Check sheet for the modelled part. Datum: model origin and axes. Units: mm. Face numbers are marked on the shaded views. A direction names the side the tool comes from. Give positions to 0.01 mm unless a question says otherwise; leave off trailing zeros. Order: outer loops, then holes, each group sorted by start corner. A loop starts at its lowest first (then second) coordinate and runs counter-clockwise, first axis right, second up.
Item 1: Sectioned sample at A-A on x = 0. Record the boundary of the cut face in (y, z), and give its area (3 significant figures).
Item 2: Material ranges on line 1 along Z through (x, y) = (-0.95, -0.6); line 2 along Z through (x, y) = (-2.05, 0.45); line 3 along X through (y, z) = (0.9, 19), recorded low to high.
Item 3: Gauge pin test, flat ends, axial feed: P1, Ø0.8, axis at x = 0, y = 0, coming from the -Z side; P2, Ø1.5, axis at x = -1, z = 7, coming from the -Y side. Record the tip position at first contact, or that the pin passes through.
Item 4: Access from +Z, -Z, +X, -X, +Y, -Y to the whole of each face (thin tool, end or side, straight path). Record for the marked faces 1 and 2.
Item 5: Sectioned sample at B-B on z = 12. Record the boundary of the cut face in (x, y).
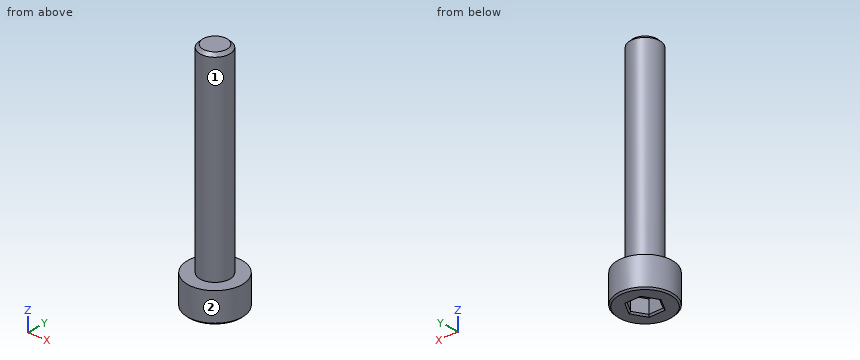
from build123d import *

# Parameters (mm, degrees)
F3_R     = 2.75
F4_DEPTH = 3
F6_DEPTH = 1.5
F7_R     = 1.5
F8_DEPTH = 20
F9_SIZE  = 0.15
F10_SIZE = 0.3


with BuildPart() as f4:
    # F3 (on Top) → F4 (new body)
    with BuildSketch(Plane.XY):
        Circle(F3_R)
    extrude(amount=F4_DEPTH)

    # F5 (on face) → F6 (cut)
    with BuildSketch(Plane(origin=(0, 0, 0), x_dir=(1, 0, 0), z_dir=(0, 0, -1))):
        Polygon((0.7216878365, 1.25), (-0.7216878365, 1.25), (-1.443375673, 0), (-0.7216878365, -1.25), (0.7216878365, -1.25), (1.443375673, 0), align=None)
    extrude(amount=-F6_DEPTH, mode=Mode.SUBTRACT)

    # F7 (on face) → F8 (join)
    with BuildSketch(Plane.XY.offset(3)):
        Circle(F7_R)
    extrude(amount=F8_DEPTH)

    # F9
    f9_edges = [f4.edges().sort_by_distance(p)[0] for p in [
        (-2.75, 0, 0),
        (0, -1.25, 0),
        (1.082532, -0.625, 0),
        (1.082532, 0.625, 0),
        (0, 1.25, 0),
        (-1.082532, -0.625, 0),
        (-1.082532, 0.625, 0),
    ]]
    chamfer(f9_edges, length=F9_SIZE)

    # F10
    f10_edges = [f4.edges().sort_by_distance(p)[0] for p in [
        (-1.5, 0, 23),
    ]]
    chamfer(f10_edges, length=F10_SIZE)


solid = f4.part
Report:
1. outline: (-2.75, 0.15) - (-2.6, 0) - (-1.4, 0) - (-1.25, 0.15) - (-1.25, 1.5) - (1.25, 1.5) - (1.25, 0.15) - (1.4, 0) - (2.6, 0) - (2.75, 0.15) - (2.75, 3) - (1.5, 3) - (1.5, 22.7) - (1.2, 23) - (-1.2, 23) - (-1.5, 22.7) - (-1.5, 3) - (-2.75, 3) - close
1. area: 72.6 mm2
2. line 1: z = 1.5 to 23
2. line 2: z = 0 to 3
2. line 3: x = -1.2 to 1.2
3. P1: stops at z = 1.5
3. P2: stops at y = -1.48
4. face 1: +Z
4. face 2: +Z, -Z
5. outline: circle Ø3 at (0, 0)
